Check sheet for the modelled part. Datum: model origin and axes. Units: mm. A direction names the side the tool comes from. Round coordinates to 2 decimals unless told otherwise and drop trailing zeros. Write each loop counter-clockwise with the first axis right and the second up, starting at its lowest first coordinate (ties: lowest second). Pieces come first, ordered by that corner, then holes.
from build123d import *

# Parameters (mm, degrees)
SKETCH1_R           = 16.3
BOSS_EXTRUDE1_DEPTH = 28
FILLET1_R           = 10
SKETCH4_R           = 5.2
SKETCH5_R           = 3.05
SKETCH6_R           = 3.05
CUT_EXTRUDE1_DEPTH  = 9
BOSS_EXTRUDE3_START = 9
BOSS_EXTRUDE3_DEPTH = 9
BOSS_EXTRUDE4_DEPTH = 10
CIRPATTERN1_COUNT   = 6
FILLET2_R           = 3


with BuildPart() as part:
    # Sketch1 → Boss-Extrude1 (new body)
    with BuildSketch(Plane(origin=(0, 0, 0), x_dir=(1, 0, 0), z_dir=(0, 1, 0))):
        with Locations(Location((0, 0, 0), (0, 0, 270))):
            Circle(SKETCH1_R)
    extrude(amount=BOSS_EXTRUDE1_DEPTH)

    # Fillet1
    fillet1_edges = [part.edges().sort_by_distance(p)[0] for p in [
        (0, 28, -16.3),
    ]]
    fillet(fillet1_edges, radius=FILLET1_R)

    # Sketch4 → Cut-Loft1 section 0
    with BuildSketch(Plane.XZ):
        Circle(SKETCH4_R)
    # Sketch5 → Cut-Loft1 section 1
    with BuildSketch(Plane(origin=(0, 7, 0), x_dir=(-1, 0, 0), z_dir=(0, -1, 0))):
        Circle(SKETCH5_R)
    loft(mode=Mode.SUBTRACT)

    # Sketch6 → Cut-Extrude1 (cut)
    with BuildSketch(Plane.XZ.offset(-7)):
        with Locations(Location((0, 0, 0), (0, 0, 270))):
            Circle(SKETCH6_R)
    extrude(amount=-CUT_EXTRUDE1_DEPTH, mode=Mode.SUBTRACT)

    # Sketch7 → Boss-Extrude3 (add)
    with BuildSketch(Plane.XZ.offset(-16).offset(BOSS_EXTRUDE3_START)):
        with BuildLine():
            Line((-2.424871131, 1.85), (2.424871131, 1.85))
            ThreePointArc((2.424871131, 1.85), (0, 3.05), (-2.424871131, 1.85))
        make_face()
    extrude(amount=-BOSS_EXTRUDE3_DEPTH)

    # Sketch8 → Boss-Extrude4 (add)
    with BuildSketch(Plane(origin=(0, 18, 0), x_dir=(-1, 0, 0), z_dir=(0, -1, 0))):
        Polygon((0, 6.3), (-2, 6.3), (-2, 16.3), (0, 16.3), (2, 16.3), (2, 6.3), align=None)
    boss_extrude4 = extrude(amount=-BOSS_EXTRUDE4_DEPTH)

    # CirPattern1: Boss-Extrude4 ×6 about axis
    cirpattern1_axis = Axis((0, 0, 0), (0, 1, 0))
    for i in range(1, CIRPATTERN1_COUNT):
        add(boss_extrude4.rotate(cirpattern1_axis, i * 360 / CIRPATTERN1_COUNT))

    # Fillet2
    fillet2_edges = [part.edges().sort_by_distance(p)[0] for p in [
        (14.116214082, 28, 8.15),
        (14.116214082, 28, -8.15),
        (0, 28, -16.3),
        (-14.116214082, 28, -8.15),
        (-14.116214082, 28, 8.15),
        (0, 28, 16.3),
    ]]
    fillet(fillet2_edges, radius=FILLET2_R)


solid = part.part
1. Sectioned sample at B-B, the plane y = 2.75. Enter the section's corners in (x, z).
2. Sectioned sample at A-A, the plane y = 11.5. Enter the section's corners in (x, z), plus the area to 3 significant figures.
3. Release check for a two-part mould opening along Z. For faces 1 (the cylindrical face through (13.36, 27.1, 7.75)), 2 (the flat face through (13.052, 25.199, 5.226)), 3 (the flat face through (-2, 26, 14)) record: released by +Z, released by -Z, zero draft, split by the parting line, or undercut.
4. Go/stop test with flat-tipped pins: pin 1 (1.1 mm diameter, centred on x = -14.5, z = 7.5, fed in from -Y); pin 2 (8 mm diameter, centred on x = -9, y = 14.5, fed in from -Z); pin 3 (5 mm diameter, centred on y = 7.5, z = 8, fed in from -X); pin 4 (1.5 mm diameter, centred on x = -2.5, y = 6, fed in from +Z). Record where each tip stops, or that it passes through.
5. Scan lines: line 1 along X through (y, z) = (12.5, 0); line 2 along Z through (x, y) = (0, 11.25); line 3 along Z through (x, y) = (-2, 13.5). Record each from-to range of solid material in increasing order.
6. Set-up check for faces 4 (the flat face through (0, 7, 2.3)), 5 (the flat face through (-11.05, 25.2, 8.69)), 6 (the cylindrical face through (-13.389, 27.098, 7.698)): record each of +Z, -Z, +X, -X, +Y, -Y from which the full face is reachable in a straight line by a thin tool's end or side.
Computed values:
1. outline: circle Ø32.6 at (0, 0); hole circle Ø8.71 at (0, 0)
2. outline: circle Ø32.6 at (0, 0); hole (-2.42, 1.85) arc R3.05 ccw (long way) to (2.42, 1.85) - close
2. area: 810 mm2
3. face 1: released by +Z
3. face 2: undercut
3. face 3: zero draft
4. pin 1: stops at y = 0
4. pin 2: stops at z = -15.51
4. pin 3: stops at x = -15.34
4. pin 4: stops at z = 16.21
5. line 1: x = -16.3 to -3.05, 3.05 to 16.3
5. line 2: z = -16.3 to -3.05, 1.85 to 16.3
5. line 3: z = -16.18 to -2.3, 1.85 to 16.18
6. face 4: -Y
6. face 5: +Z, +Y
6. face 6: +Z, -X, +Y
